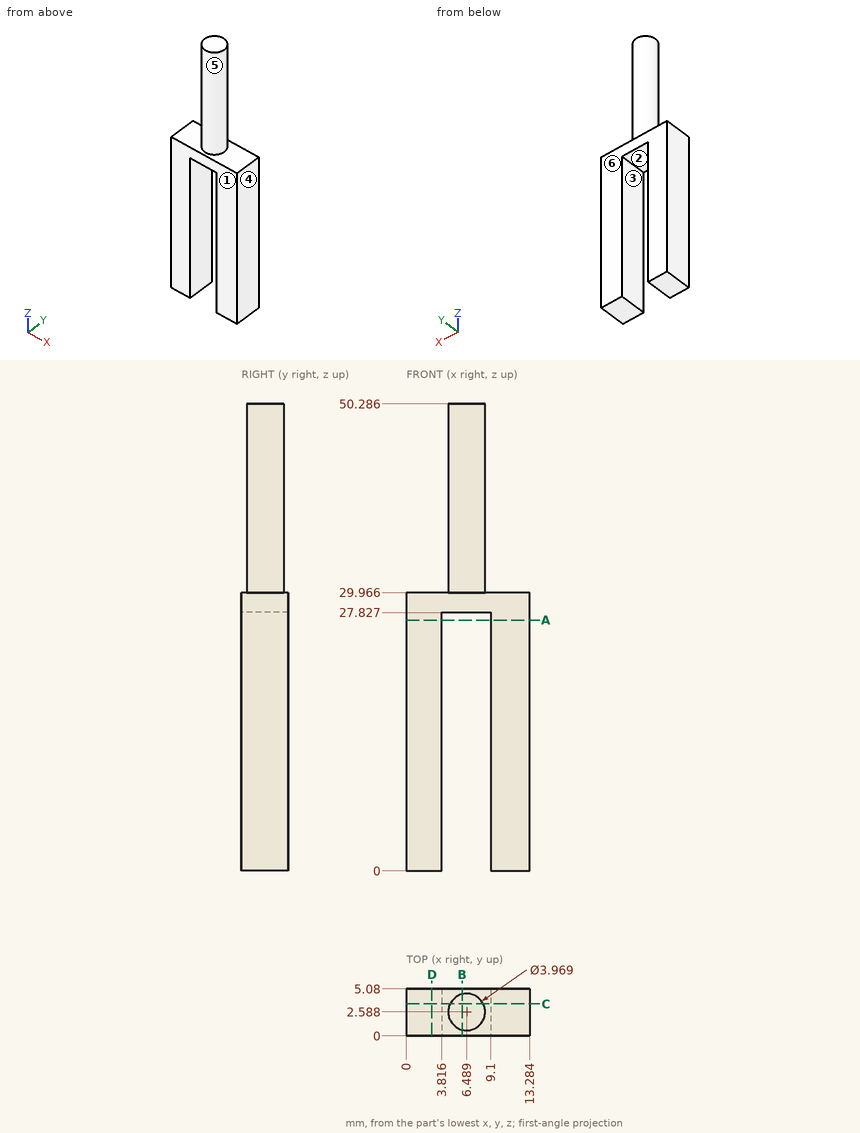
Could you check a few things on this drawing? It's one solid part, dimensions in mm from its lowest x, y, z. A direction names the side the tool comes from. Coordinates: 2 decimals unless noted, no trailing zeros. Order: outer loops, then holes, each group sorted by start corner. A loop starts at its lowest first (then second) coordinate and runs counter-clockwise, first axis right, second up. Notation, with made-up numbers: (-27.5, 53.5) -> (28.5, 53.5) arc R24 cw to (28.5, 78.5) -> close; hole circle Ø3 at (-18.75, 71). An arc over 180 degrees is marked (long way). Answer in a Markdown table with one row per item.
(1) I want a section at C-C on y = 3.45. List the corners of the cut face in (x, z) for me.
Answer key:
| item | result |
|---|---|
| outline | (0, 0) -> (3.82, 0) -> (3.82, 27.83) -> (9.1, 27.83) -> (9.1, 0) -> (13.28, 0) -> (13.28, 29.97) -> (8.28, 29.97) -> (8.28, 50.29) -> (4.7, 50.29) -> (4.7, 29.97) -> (0, 29.97) -> close |
(2) Please list where these lines run through material, in increasing order: probe 1 along X at (y, z) = (2.15, 20.5); probe 2 along Z at (x, y) = (3.5, 2.25); probe 3 along Z at (x, y) = (4.25, 2.15).
Answer key:
| item | result |
|---|---|
| probe 1 | 0 to 3.82, 9.1 to 13.28 |
| probe 2 | 0 to 29.97 |
| probe 3 | 27.83 to 29.97 |
(3) On a 3-axis mill with a long thin cutter (end or side, diameter ignored), from which of +Z, -Z, +X, -X, +Y, -Y can I reach the whole of each face in a straight line? I mean the marked faces 1 and 2. Say none if no direction works.
Answer key:
| item | result |
|---|---|
| face 1 | +Z, -Z, +X, -X, -Y |
| face 2 | -Z, +Y, -Y |
(4) I want a section at D-D on x = 2.75. List the corners of the cut face in (y, z) for me, then the cut area to 3 significant figures.
Answer key:
| item | result |
|---|---|
| outline | (0, 0) -> (5.08, 0) -> (5.08, 29.97) -> (0, 29.97) -> close |
| area | 152 mm^2 |
(5) I want a section at A-A on z = 27. List the corners of the cut face in (x, y) for me.
Answer key:
| item | result |
|---|---|
| outline | (0, 0) -> (3.82, 0) -> (3.82, 5.08) -> (0, 5.08) -> close; (9.1, 0) -> (13.28, 0) -> (13.28, 5.08) -> (9.1, 5.08) -> close |
(6) Thinking about a two-plate mould opening in X: for the marked faces 3, 4, 5 and 6, which applies, +X half, -X half, draft (parallel to the pull), parting line (faces both ways), or undercut?
Answer key:
| item | result |
|---|---|
| face 3 | undercut |
| face 4 | +X half |
| face 5 | parting line |
| face 6 | draft |
(7) I want a section at B-B on x = 6. List the corners of the cut face in (y, z) for me (1 decimal).
Answer key:
| item | result |
|---|---|
| outline | (0, 27.8) -> (5.1, 27.8) -> (5.1, 30) -> (4.5, 30) -> (4.5, 50.3) -> (0.7, 50.3) -> (0.7, 30) -> (0, 30) -> close |
